from build123d import *

# Parameters (mm, degrees)
SKETCH1_W            = 65
SKETCH1_H            = 55
BOSS_EXTRUDE1_DEPTH  = 5
SKETCH2_R            = 1.5
CUT_EXTRUDE1_DEPTH   = 5
SKETCH3_R            = 3.25
CUT_EXTRUDE2_DEPTH   = 2
LPATTERN1_COUNT      = 2
LPATTERN1_PITCH      = 20
LPATTERN1_COUNT_DIR2 = 3
LPATTERN1_PITCH_DIR2 = 20
SKETCH5_W            = 35
SKETCH5_H            = 5
BOSS_EXTRUDE2_DEPTH  = 35
SKETCH6_R            = 1.25
CUT_EXTRUDE3_DEPTH   = 35


with BuildPart() as part:
    # Sketch1 → Boss-Extrude1 (new body)
    with BuildSketch(Plane(origin=(0, 0, 0), x_dir=(1, 0, 0), z_dir=(0, 1, 0))):
        Rectangle(SKETCH1_W, SKETCH1_H)
    extrude(amount=BOSS_EXTRUDE1_DEPTH)

    # Sketch2 → Cut-Extrude1 (cut)
    with BuildSketch(Plane(origin=(0, 5, 0), x_dir=(1, 0, 0), z_dir=(0, 1, 0))):
        with Locations(Location((-20, 10, 0), (0, 0, 270))):
            Circle(SKETCH2_R)
        with Locations(Location((0, 10, 0), (0, 0, 270))):
            Circle(SKETCH2_R)
        with Locations(Location((20, 10, 0), (0, 0, 270))):
            Circle(SKETCH2_R)
        with Locations(Location((-20, -10, 0), (0, 0, 270))):
            Circle(SKETCH2_R)
        with Locations(Location((0, -10, 0), (0, 0, 270))):
            Circle(SKETCH2_R)
        with Locations(Location((20, -10, 0), (0, 0, 270))):
            Circle(SKETCH2_R)
    extrude(amount=-CUT_EXTRUDE1_DEPTH, mode=Mode.SUBTRACT)

    # Sketch3 → Cut-Extrude2 (cut)
    with BuildSketch(Plane(origin=(0, 5, 0), x_dir=(1, 0, 0), z_dir=(0, 1, 0))):
        with Locations(Location((-20, 10, 0), (0, 0, 270))):
            Circle(SKETCH3_R)
    cut_extrude2 = extrude(amount=-CUT_EXTRUDE2_DEPTH, mode=Mode.SUBTRACT)

    # LPattern1: Cut-Extrude2 2 × 3
    with Locations(*[(j * LPATTERN1_PITCH_DIR2, 0, i * LPATTERN1_PITCH) for i in range(LPATTERN1_COUNT) for j in range(LPATTERN1_COUNT_DIR2) if (i, j) != (0, 0)]):
        add(cut_extrude2, mode=Mode.SUBTRACT)

    # Sketch5 → Boss-Extrude2 (add)
    with BuildSketch(Plane(origin=(0, 5, 0), x_dir=(1, 0, 0), z_dir=(0, 1, 0))):
        with Locations((15, -25)):
            Rectangle(SKETCH5_W, SKETCH5_H)
    extrude(amount=BOSS_EXTRUDE2_DEPTH)

    # Sketch6 → Cut-Extrude3 (cut)
    with BuildSketch(Plane.XY.offset(27.5)):
        with Locations((4.055342901, 32)):
            Circle(SKETCH6_R)
        with Locations((4.055342901, 8)):
            Circle(SKETCH6_R)
        with Locations((28.055342901, 32)):
            Circle(SKETCH6_R)
        with Locations((28.055342901, 8)):
            Circle(SKETCH6_R)
    extrude(amount=-CUT_EXTRUDE3_DEPTH, mode=Mode.SUBTRACT)


solid = part.part
Can you work these out from the model? Positions are in its coordinate system, mm. A direction names the side the tool comes from. Coordinates: 2 decimals unless noted, no trailing zeros. Write each loop counter-clockwise with the first axis right and the second up, starting at its lowest first coordinate (ties: lowest second). Pieces come first, ordered by that corner, then holes. Notation, with made-up numbers: M 26.5,-10.75 L 50.5,-10.75 A26 cw 50.5,7.25 Z; hole C -22.5,47 d9. An arc over 180 degrees is marked long. Use one line per item in the form item = value.
Q1. If we section it at C-C (x = 0): Write out the boundary of the cut face in (y, z), then the cut area to 3 significant figures.
Model answer:
outline = M 0,-27.5 L 5,-27.5 L 5,-13.25 L 3,-13.25 L 3,-11.5 L 0,-11.5 Z; M 0,-8.5 L 3,-8.5 L 3,-6.75 L 5,-6.75 L 5,6.75 L 3,6.75 L 3,8.5 L 0,8.5 Z; M 0,11.5 L 3,11.5 L 3,13.25 L 5,13.25 L 5,22.5 L 40,22.5 L 40,27.5 L 0,27.5 Z
area = 406 mm^2
Q2. We'd pull the mould along Y, two halves only. Please class faces 4 (the flat face through (14, 20, 27.5)), 5 (the flat face through (15, 40, 25)), 6 (the cylindrical face through (3.78, 6.78, 25.04)): +Y half, -Y half, draft (parallel to the pull), parting line (faces both ways), or undercut.
Model answer:
face_4 = draft
face_5 = +Y half
face_6 = undercut
Q3. If we section it at A-A (y = 32): Write out the boundary of the cut face in (x, z).
Model answer:
outline = M -2.5,22.5 L 2.81,22.5 L 2.81,27.5 L -2.5,27.5 Z; M 5.31,22.5 L 26.81,22.5 L 26.81,27.5 L 5.31,27.5 Z; M 29.31,22.5 L 32.5,22.5 L 32.5,27.5 L 29.31,27.5 Z
Q4. I need wall thicknesses on line 1 along X through (y, z) = (1.5, -10); line 2 along X through (y, z) = (3.4, 10); line 3 along Z through (x, y) = (12.5, 22). Which ranges of each line are inside material? Lowest first, please. Write a range as from..to.
Model answer:
line_1 = -32.5..-21.5, -18.5..-1.5, 1.5..18.5, 21.5..32.5
line_2 = -32.5..-23.25, -16.75..-3.25, 3.25..16.75, 23.25..32.5
line_3 = 22.5..27.5
Q5. For faces 1 (the cylindrical face through (0.07, 1.52, 8.5)), 2 (the flat face through (15, 22, 22.5)), 3 (the flat face through (21.5, 3, -9.3)), which set-ups out of +Z, -Z, +X, -X, +Y, -Y let a thin tool reach every point of the face, with its end or its side?
Model answer:
face_1 = +Y, -Y
face_2 = -Z, +X, -X, +Y
face_3 = +Y
Q6. For P1, Ø1.8, axis at x = -20, z = 10, coming from the -Y side; P2, Ø10, axis at x = 24.5, y = 16.5, coming from the -Z side; P3, Ø7, axis at x = -18.5, z = 11, coming from the +Y side; P4, Ø5, axis at x = 0, z = -10, coming from the +Y side, each with a flat end and sliding along its axis, tell me the tip position at first contact or that it passes through.
Model answer:
P1 = through
P2 = 22.5
P3 = 5
P4 = 3
Q7. If we section it at D-D (z = 24): Write out the boundary of the cut face in (x, y).
Model answer:
outline = M -32.5,0 L 32.5,0 L 32.5,40 L -2.5,40 L -2.5,5 L -32.5,5 Z; hole C 4.06,8 d2.5; hole C 4.06,32 d2.5; hole C 28.06,8 d2.5; hole C 28.06,32 d2.5
Q8. If we section it at B-B (z = 10): Write out the boundary of the cut face in (x, y).
Model answer:
outline = M -32.5,0 L -21.5,0 L -21.5,3 L -23.25,3 L -23.25,5 L -32.5,5 Z; M -18.5,0 L -1.5,0 L -1.5,3 L -3.25,3 L -3.25,5 L -16.75,5 L -16.75,3 L -18.5,3 Z; M 1.5,0 L 18.5,0 L 18.5,3 L 16.75,3 L 16.75,5 L 3.25,5 L 3.25,3 L 1.5,3 Z; M 21.5,0 L 32.5,0 L 32.5,5 L 23.25,5 L 23.25,3 L 21.5,3 Z
